```python
from build123d import *

# Parameters (mm, degrees)
F0_R     = 10.5
F0_R_2   = 6
F1_DEPTH = 30
F2_R     = 0.25
F4_START = -3.5
F3_R     = 16
F3_R_2   = 10
F4_DEPTH = 1.3
F5_START = -25.2
F5_DEPTH = 1.3


with BuildPart() as f1:
    # F0 (on Top) → F1 (new body)
    with BuildSketch(Plane.XY):
        Circle(F0_R)
        Circle(F0_R_2, mode=Mode.SUBTRACT)
    extrude(amount=F1_DEPTH)

    # F2
    f2_edges = [f1.edges().sort_by_distance(p)[0] for p in [
        (-10.5, 0, 30),
        (-6, 0, 30),
        (-10.5, 0, 0),
        (-6, 0, 0),
    ]]
    fillet(f2_edges, radius=F2_R)

    # F3 (on face) → F4 (cut)
    with BuildSketch(Plane.XY.offset(30).offset(F4_START)):
        Circle(F3_R)
        Circle(F3_R_2, mode=Mode.SUBTRACT)
    extrude(amount=-F4_DEPTH, mode=Mode.SUBTRACT)

    # F3 (on face) → F5 (cut)
    with BuildSketch(Plane.XY.offset(30).offset(F5_START)):
        Circle(F3_R)
        Circle(F3_R_2, mode=Mode.SUBTRACT)
    extrude(amount=-F5_DEPTH, mode=Mode.SUBTRACT)


solid = f1.part
```
Work out the finished part from the listing and answer in its coordinate system (mm). A direction names the side the tool comes from. Round coordinates to 2 decimals unless told otherwise and drop trailing zeros. Loops run counter-clockwise (first coordinate to the right, second up) from the corner with the lowest first, then second, coordinate; pieces in that order, holes last.
(1) Find the intervals of material crossed by L1, parallel to Y at x = 0, z = 22.75; L2, parallel to X at y = 2.25, z = 2; L3, parallel to Y at x = -2.5, z = 27.5, in increasing order.
Computed values:
L1: y = -10.5 to -6, 6 to 10.5
L2: x = -10.26 to -5.56, 5.56 to 10.26
L3: y = -10.2 to -5.45, 5.45 to 10.2
(2) For faces 4 (the flat face through (5, -9, 25.2)), 5 (the flat face through (4, 5, 0)), determine the directions among +Z, -Z, +X, -X, +Y, -Y from which every point of the face is accessible in a straight line to the end or side of a thin tool.
Computed values:
face 4: none
face 5: -Z, +X, -X, +Y, -Y
(3) The part is cut by section C-C, the plane z = 4. Give the vertices of the cut face in (x, y), and give its area (3 significant figures).
Computed values:
outline: circle Ø20 at (0, 0); hole circle Ø12 at (0, 0)
area: 201 mm2
(4) Each of these flat-tipped pins is pushed along its axis until it touches: P1, Ø5, axis at x = -2.5, y = 3.5, coming from the +Z side; P2, Ø1, axis at y = -2, z = 21.5, coming from the +X side; P3, Ø1, axis at x = 1, z = 22.5, coming from the -Y side; P4, Ø8, axis at x = -7, z = 18.5, coming from the +Y side. Where does it stop, or does it pass through?
Computed values:
P1: stops at z = 30
P2: stops at x = 10.39
P3: stops at y = -10.49
P4: stops at y = 10.06
(5) The mould has two halves that part along Y. Classify faces 1 (the flat face through (5, -9, 4.8)), 2 (the cylindrical face through (-6, 0, 15)), 3 (the cylindrical face through (-2.17, -9.76, 25.86)): pulls with the +Y half, pulls with the -Y half, needs draft (parallel to the pull), parting line crosses it, or undercut.
Computed values:
face 1: needs draft
face 2: undercut
face 3: parting line crosses it
(6) The part is cut by section B-B, the plane z = 20.5. Give the vertices of the cut face in (x, y).
Computed values:
outline: circle Ø21 at (0, 0); hole circle Ø12 at (0, 0)
